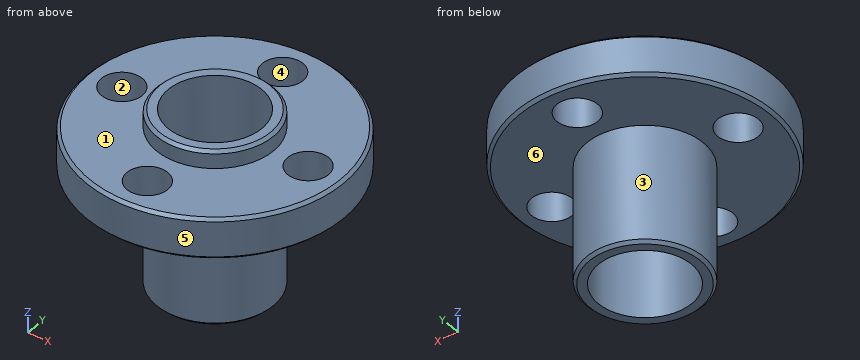
```python
from build123d import *

# Parameters (mm, degrees)
CHAMFER1_SIZE      = 0.25
CUT_EXTRUDE1_REACH = 15.5
SKETCH2_R          = 1.75


with BuildPart() as part:
    # Sketch1 → Revolve1 (revolve)
    with BuildSketch(Plane(origin=(0, 0, 0), x_dir=(0, 0, -1), z_dir=(1, 0, 0))):
        Polygon((0, 4), (15, 4), (15, 5), (5, 5), (5, 11), (1.5, 11), (1.5, 5), (0, 5), align=None)
    revolve(axis=Axis((0, 0, 903.973270396), (0, 0, -1)))

    # Chamfer1
    chamfer1_edges = [part.edges().sort_by_distance(p)[0] for p in [
        (0, -5, 0),
        (0, -11, -1.5),
        (0, -11, -5),
        (0, -5, -15),
    ]]
    chamfer(chamfer1_edges, length=CHAMFER1_SIZE)

    # Sketch2 → Cut-Extrude1 (cut, up to next)
    with BuildSketch(Plane.XY.offset(-1.5), mode=Mode.PRIVATE) as cut_extrude1_sk1:
        with Locations((0, 8)):
            Circle(SKETCH2_R)
    cut_extrude1_tool1 = extrude(cut_extrude1_sk1.sketch, amount=-CUT_EXTRUDE1_REACH, mode=Mode.PRIVATE) & part.part
    add(cut_extrude1_tool1.solids().sort_by_distance((0, 8, -1.5))[0], mode=Mode.SUBTRACT)
    # Sketch2 → Cut-Extrude1 (cut, up to next)
    with BuildSketch(Plane.XY.offset(-1.5), mode=Mode.PRIVATE) as cut_extrude1_sk2:
        with Locations((8, 0)):
            Circle(SKETCH2_R)
    cut_extrude1_tool2 = extrude(cut_extrude1_sk2.sketch, amount=-CUT_EXTRUDE1_REACH, mode=Mode.PRIVATE) & part.part
    add(cut_extrude1_tool2.solids().sort_by_distance((8, 0, -1.5))[0], mode=Mode.SUBTRACT)
    # Sketch2 → Cut-Extrude1 (cut, up to next)
    with BuildSketch(Plane.XY.offset(-1.5), mode=Mode.PRIVATE) as cut_extrude1_sk3:
        with Locations((0, -8)):
            Circle(SKETCH2_R)
    cut_extrude1_tool3 = extrude(cut_extrude1_sk3.sketch, amount=-CUT_EXTRUDE1_REACH, mode=Mode.PRIVATE) & part.part
    add(cut_extrude1_tool3.solids().sort_by_distance((0, -8, -1.5))[0], mode=Mode.SUBTRACT)
    # Sketch2 → Cut-Extrude1 (cut, up to next)
    with BuildSketch(Plane.XY.offset(-1.5), mode=Mode.PRIVATE) as cut_extrude1_sk4:
        with Locations((-8, 0)):
            Circle(SKETCH2_R)
    cut_extrude1_tool4 = extrude(cut_extrude1_sk4.sketch, amount=-CUT_EXTRUDE1_REACH, mode=Mode.PRIVATE) & part.part
    add(cut_extrude1_tool4.solids().sort_by_distance((-8, 0, -1.5))[0], mode=Mode.SUBTRACT)


solid = part.part
```
Design review of the part built by this model. Coordinates are the model's own, in mm. Face numbers are marked on the shaded views. A direction names the side the tool comes from. Give positions to 0.01 mm unless a question says otherwise; leave off trailing zeros. Loops run counter-clockwise (first coordinate to the right, second up) from the corner with the lowest first, then second, coordinate; pieces in that order, holes last. Notation, with made-up numbers: (68, -19.75) -> (74, -19.75) arc R17 ccw to (74, 0.25) -> close; hole circle Ø9 at (22.5, 88). An arc over 180 degrees is marked (long way). One line per item, written item: value.
Q1. We need section A-A on x = 0. Give the number of separate pieces and of enclosed holes in the cut face, and give its area (4 significant figures).
Numbers:
separate pieces: 4
enclosed holes: 0
area: 47.25 mm^2
Q2. Machinability: for the marked faces 1, 2 and 3, which of the approach directions +Z, -Z, +X, -X, +Y, -Y give a long, thin tool a straight path to every point of the face, cutting with its end or side? Answer none if there is none.
Numbers:
face 1: +Z
face 2: +Z, -Z
face 3: -Z
Q3. Draft analysis for pull direction Y (two halves, no side actions). For the marked faces 4, 5 and 6, state which applies: pulls with the +Y half, pulls with the -Y half, needs draft (parallel to the pull), parting line crosses it, or undercut.
Numbers:
face 4: undercut
face 5: parting line crosses it
face 6: needs draft
Q4. For L1, parallel to X at y = 0.25, z = -3.25; L2, parallel to X at y = 0, z = -7.75; L3, parallel to Z at x = 5.5, y = 6.25, list the stretches that pass through material, from the lowest coordinate up.
Numbers:
L1: x = -11 to -9.73, -6.27 to -3.99, 3.99 to 6.27, 9.73 to 11
L2: x = -5 to -4, 4 to 5
L3: z = -5 to -1.5
Q5. We need section B-B on z = -10.5. Give the boundary of the cut face in (x, y), and give its area (3 significant figures).
Numbers:
outline: circle Ø10 at (0, 0); hole circle Ø8 at (0, 0)
area: 28.3 mm^2
Q6. For pin 1 Ø5 at (x, y) = (4.5, -6.5) entering from -Z; pin 2 Ø1.5 at (x, y) = (4.5, 3.5) entering from +Z; pin 3 Ø1 at (y, z) = (-0.5, -7.5) entering from +X, all flat-tipped, find the tip position at first contact; note any pin that passes through.
Numbers:
pin 1: stops at z = -5
pin 2: stops at z = -0.2
pin 3: stops at x = 5
